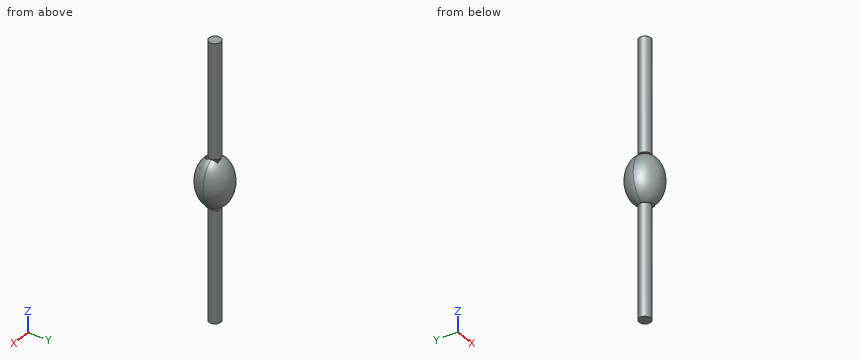
Autodesk Inventor part; units mm, degrees
ref_plane "Work Plane2" through (0, 0, -100) normal (0, 0, 1) x (1, 0, 0)
ref_plane "Work Plane3" through (0, 0, 100) normal (0, 0, 1) x (1, 0, 0)
ref_plane "YZ Plane" through (0, 0, 0) normal (1, 0, 0) x (0, 1, 0)
sketch "Sketch3" plane through (0, 0, 0) normal (0, 1, 0) x (-1, 0, 0)
  ellipse E0 centre (0, 0) end of major axis (0, 100) minor radius 70.1032
  line L0 (0, 100) -> (0, -100)
  dimension "d6" = 100
revolve "Revolution2" add sketch "Sketch3" angle 360 about axis through (0, 0, 100) along (0, 0, -1) picked at (-23.3548, 1.1091) contours L0 E0
ref_plane "Work Plane2" through (0, 0, -100) normal (0, 0, 1) x (1, 0, 0)
sketch "Sketch4" plane through (0, 0, -100) normal (0, 0, 1) x (1, 0, 0)
  line L0 (70.1032, 0) -> (0, 0)
  circle A0 centre (0, 0) radius 23.8125
  dimension "d9" = 47.625
extrude "Extrusion1" add sketch "Sketch4" against normal blind 406.515
ref_plane "Work Plane3" through (0, 0, 100) normal (0, 0, 1) x (1, 0, 0)
sketch "Sketch5" plane through (0, 0, 100) normal (0, 0, 1) x (1, 0, 0)
  line L0 (70.1032, 0) -> (0, 0)
  circle A0 centre (0, 0) radius 23.8125
  point P0 (23.8125, 0)
extrude "Extrusion2" add sketch "Sketch5" along normal blind 406.515
sketch "Sketch6" plane through (0, 0, -506.515) normal (0, 0, -1) x (-1, 0, 0)
  circle A0 centre (0, 0) radius 23.8125
extrude "Extrusion3" add sketch "Sketch6" along normal blind 46.103
sketch "Sketch7" plane through (0, 0, 506.515) normal (0, 0, 1) x (1, 0, 0)
  circle A0 centre (0, 0) radius 23.8125
extrude "Extrusion4" add sketch "Sketch7" along normal blind 46.103
sketch "Sketch8" plane through (0, 0, 552.618) normal (0, 0, 1) x (1, 0, 0)
  circle A0 centre (0, 0) radius 23.8125
extrude "Extrusion5" add sketch "Sketch8" along normal blind 7.794
sketch "Sketch9" plane through (0, 0, 0) normal (1, 0, 0) x (0, 1, 0)
  line L0 (-23.8125, -100) -> (23.8125, -100)
  line L1 (-23.8125, 100) -> (23.8125, 100)
  line L2 (-23.8125, -100) -> (23.8125, -100)
  line L3 (23.8125, -100) -> (23.8125, 100)
  line L4 (23.8125, 100) -> (-23.8125, 100)
  line L5 (-23.8125, 100) -> (-23.8125, -100)
  point P0 (0, 0)
extrude "Extrusion6" add sketch "Sketch9" along normal blind 20
properties part number "Differential"
Read the model definition and answer for the solid it produces. Units are mm, in the model's axes. Give positions to 0.01 mm unless a question says otherwise; leave off trailing zeros. Write each loop counter-clockwise with the first axis right and the second up, starting at its lowest first coordinate (ties: lowest second). Pieces come first, ordered by that corner, then holes. Notation, with made-up numbers: M 31,19 L 50,19 A14 ccw 50,27 Z; hole C 26.5,-26 d9. An arc over 180 degrees is marked long. Put each result on its own line as item: value. Start each with the question number.
1. Consider line 1 along Y through (x, z) = (2, 400.5); line 2 along Z through (x, y) = (17.5, -23); line 3 along Y through (x, z) = (3, 60). Determine where each line is inside the solid, lowest interval first.
2. The part is cut by section A-A, the plane z = 269.5. Give the vertices of the cut face in (x, y) (1 decimal).
3. Each of these flat-tipped pins is pushed along its axis until it touches: pin 1 Ø8 at (y, z) = (-8, 167) entering from +X; pin 2 Ø11.5 at (y, z) = (9.5, -92.5) entering from +X; pin 3 Ø4 at (x, z) = (-20, 27.5) entering from -Y; pin 4 Ø3.5 at (x, y) = (15, -20) entering from +Z. Where does it stop, or does it pass through?
Final values:
1. line 1: y = -23.73 to 23.73
1. line 2: z = -100 to 100
1. line 3: y = -56 to 56
2. outline: C 0,0 d47.6
3. pin 1: stops at x = 23.47
3. pin 2: stops at x = 33.71
3. pin 3: stops at y = -65.08
3. pin 4: stops at z = 560.41
